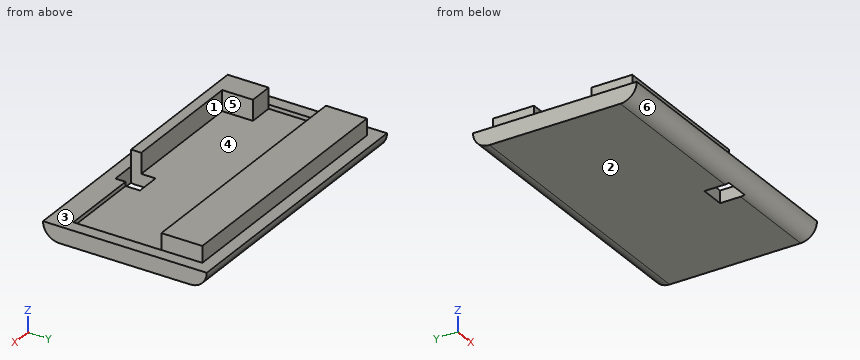
```python
from build123d import *

# Parameters (mm, degrees)
SKETCH1_W           = 34.5
SKETCH1_H           = 20
BOSS_EXTRUDE1_DEPTH = 2
SKETCH2_W           = 31.5
SKETCH2_H           = 5
BOSS_EXTRUDE2_DEPTH = 2
SKETCH3_W           = 3
SKETCH3_H           = 3
CUT_EXTRUDE1_DEPTH  = 10
FILLET1_R           = 2
CUT_EXTRUDE2_DEPTH  = 2
CUT_EXTRUDE3_DEPTH  = 2.5


with BuildPart() as part:
    # Sketch1 → Boss-Extrude1 (new body)
    with BuildSketch(Plane.XY):
        Rectangle(SKETCH1_W, SKETCH1_H)
    extrude(amount=BOSS_EXTRUDE1_DEPTH)

    # Sketch2 → Boss-Extrude2 (add)
    with BuildSketch(Plane.XY.offset(2)):
        with Locations((0, 6)):
            Rectangle(SKETCH2_W, SKETCH2_H)
        with Locations((0, -6)):
            Rectangle(SKETCH2_W, SKETCH2_H)
    extrude(amount=BOSS_EXTRUDE2_DEPTH)

    # Sketch3 → Cut-Extrude1 (cut)
    with BuildSketch(Plane(origin=(0, 0, 0), x_dir=(-1, 0, 0), z_dir=(0, 0, -1))):
        with Locations((-4.25, -7)):
            Rectangle(SKETCH3_W, SKETCH3_H)
    extrude(amount=-CUT_EXTRUDE1_DEPTH, mode=Mode.SUBTRACT)

    # Fillet1
    # the kernel refuses this fillet: 2 mm, written as the material it takes off along each edge
    with BuildSketch(Plane(origin=(22.25, -10, 0), x_dir=(0, 1, 0), z_dir=(-1, 0, 0))) as fillet1_piece_1:
        with BuildLine():
            CenterArc((FILLET1_R, -FILLET1_R), FILLET1_R, 90, 90)
            Line((0, -FILLET1_R), (0, 0))
            Line((0, 0), (FILLET1_R, 0))
        make_face()
    extrude(amount=44.5, mode=Mode.SUBTRACT)
    with BuildSketch(Plane(origin=(-22.25, 10, 0), x_dir=(0, 0, 1), z_dir=(1, 0, 0))) as fillet1_piece_2:
        with BuildLine():
            CenterArc((FILLET1_R, FILLET1_R), FILLET1_R, 180, 90)
            Line((0, FILLET1_R), (0, 0))
            Line((0, 0), (FILLET1_R, 0))
        make_face()
    extrude(amount=44.5, mode=Mode.SUBTRACT)

    # Sketch4 → Cut-Extrude2 (cut)
    with BuildSketch(Plane.XY.offset(4)):
        Polygon((15.75, -8.5), (5.75, -8.5), (5.75, -5.5), (-12.75, -5.5), (-12.75, -3.5), (5.75, -3.5), (15.75, -3.5), align=None)
    extrude(amount=-CUT_EXTRUDE2_DEPTH, mode=Mode.SUBTRACT)

    # Sketch6 → Cut-Extrude3 (cut)
    with BuildSketch(Plane.XY.offset(4)):
        Polygon((-15.75, 3.5), (15.762886562, 3.5), (15.762886562, -7.25), (-12.75, -7.25), (-12.75, -3.5), (-15.75, -3.5), align=None)
    extrude(amount=-CUT_EXTRUDE3_DEPTH, mode=Mode.SUBTRACT)


solid = part.part
```
The listing builds one solid part. Answer for the finished solid, in the listing's coordinates (mm). Face numbers are marked on the shaded views. A direction names the side the tool comes from. Coordinates: 2 decimals unless noted, no trailing zeros. Write each loop counter-clockwise with the first axis right and the second up, starting at its lowest first coordinate (ties: lowest second). Pieces come first, ordered by that corner, then holes. Notation, with made-up numbers: (28.5, 0) - (84.5, 0) arc R24 cw to (84.5, 26) - close; hole circle Ø7 at (12.5, 6.5). An arc over 180 degrees is marked (long way). Return JSON: item names as keys, results as strings. Group by question number.
Q1. Which of the six approach directions +Z, -Z, +X, -X, +Y, -Y give full straight-line access (tool end or side, diameter ignored) to the marked faces 1 and 2?
Q2. For a pull along Y with two mould halves and no side action, classify the marked faces 3, 4, 5 and 6 as +Y half, -Y half, draft (parallel to the pull), parting line (faces both ways), or undercut.
Q3. The part is cut by section D-D on z = 0.55. Write down the section's boundary in (x, y).
Q4. The part is cut by section A-A on z = 3.6. Write down the section's boundary in (x, y), and give its area (3 significant figures).
Q5. The part is cut by section C-C on y = -2.5. Write down the section's boundary in (x, z), and give its area (3 significant figures).
Q6. The part is cut by section B-B on x = 8. Write down the section's boundary in (y, z).
Q7. Find the intervals of material crossed by line 1 along Y through (x, z) = (2.5, 3.65); line 2 along X through (y, z) = (-1, 1.9); line 3 along Y through (x, z) = (-15.5, 3), in increasing order. Write a range as [from, to].
Q8. Flat-ended cylindrical pins translate along their axes: pin 1 Ø1.5 at (x, y) = (1, 0.5) entering from -Z; pin 2 Ø1.6 at (y, z) = (6, 3) entering from +X; pin 3 Ø3 at (x, y) = (-3, -2) entering from +Z; pin 4 Ø1.6 at (x, z) = (0, 3) entering from +Y. Find the tip coordinate at first contact, or state that the pin passes through.
Evaluation:
{
 "1": {"face 1": "+Z", "face 2": "-Z, +X, -X, +Y, -Y"},
 "2": {"face 3": "draft", "face 4": "undercut", "face 5": "undercut", "face 6": "-Y half"},
 "3": {"outline": "(-17.25, -9.38) - (17.25, -9.38) - (17.25, 9.38) - (-17.25, 9.38) - close; hole (2.75, -8.5) - (5.75, -8.5) - (5.75, -5.5) - (2.75, -5.5) - close"},
 "4": {"outline": "(-15.75, -8.5) - (2.75, -8.5) - (2.75, -7.25) - (-12.75, -7.25) - (-12.75, -3.5) - (-15.75, -3.5) - close; (-15.75, 3.5) - (15.75, 3.5) - (15.75, 8.5) - (-15.75, 8.5) - close", "area": "192 mm2"},
 "5": {"outline": "(-17.25, 0) - (17.25, 0) - (17.25, 2) - (15.76, 2) - (15.76, 1.5) - (-15.75, 1.5) - (-15.75, 2) - (-17.25, 2) - close", "area": "53.2 mm2"},
 "6": {"outline": "(-10, 2) arc R2 ccw to (-8, 0) - (8, 0) arc R2 ccw to (10, 2) - (8.5, 2) - (8.5, 4) - (3.5, 4) - (3.5, 1.5) - (-7.25, 1.5) - (-7.25, 2) - close"},
 "7": {"line 1": "y = [-8.5, -7.25], [3.5, 8.5]", "line 2": "x = [-17.25, -15.75], [15.76, 17.25]", "line 3": "y = [-8.5, -3.5], [3.5, 8.5]"},
 "8": {"pin 1": "stops at z = 0", "pin 2": "stops at x = 15.75", "pin 3": "stops at z = 1.5", "pin 4": "stops at y = 8.5"}
}
